Geometry check sheet. Reference: drawing and pictorial views, mm from the part's lowest x, y, z. Round coordinates to 2 decimals unless told otherwise and drop trailing zeros. Write each loop counter-clockwise with the first axis right and the second up, starting at its lowest first coordinate (ties: lowest second). Pieces come first, ordered by that corner, then holes. Notation, with made-up numbers: (78, -2) - (100, -2) arc R15 cw to (100, 13) - close; hole circle Ø10 at (88, -40). An arc over 180 degrees is marked (long way). Return JSON: item names as keys, results as strings.
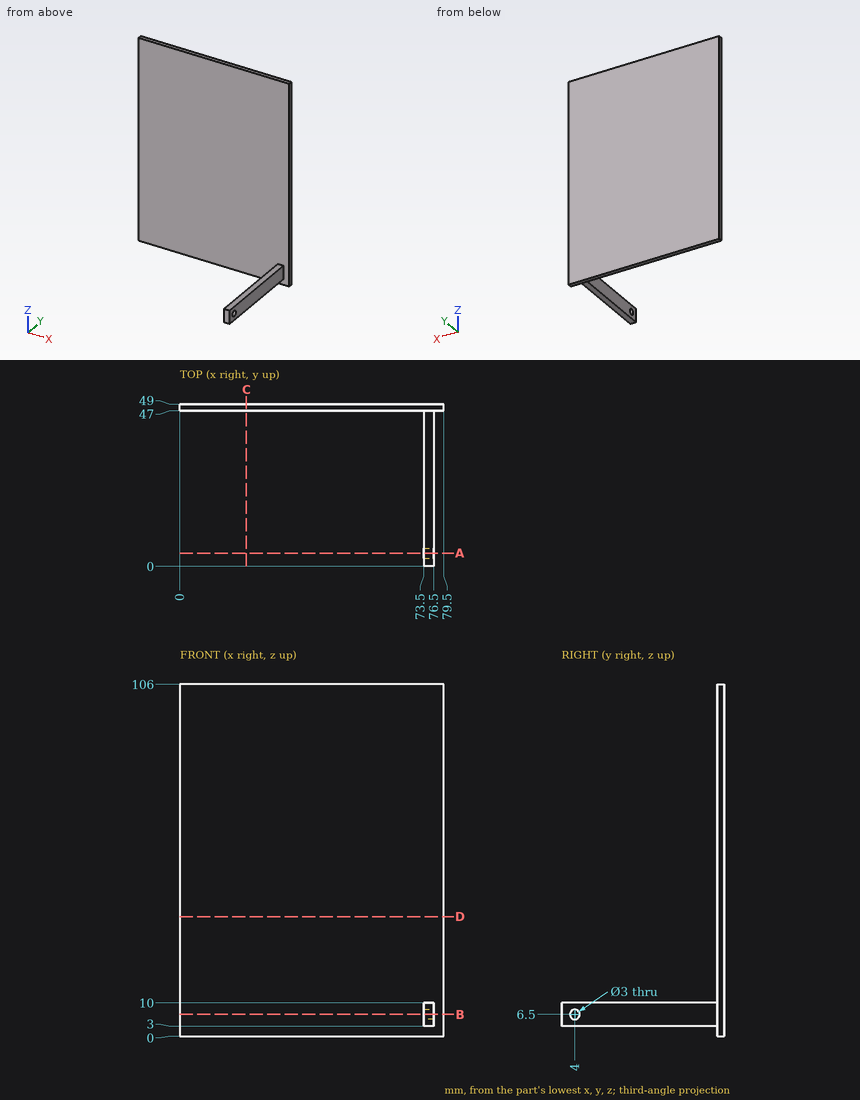
(1) Section check A-A, the plane y = 4. Enter the section's corners in (x, z), plus the area to 3 significant figures.
Response values:
{"outline": "(73.5, 3) - (76.5, 3) - (76.5, 5) - (73.5, 5) - close; (73.5, 8) - (76.5, 8) - (76.5, 10) - (73.5, 10) - close", "area": "12.0 mm^2"}
(2) Section check D-D, the plane z = 36. Enter the section's corners in (x, y).
Response values:
{"outline": "(0, 47) - (79.5, 47) - (79.5, 49) - (0, 49) - close"}
(3) Section check C-C, the plane x = 20. Enter the section's corners in (y, z), plus the area to 3 significant figures.
Response values:
{"outline": "(47, 0) - (49, 0) - (49, 106) - (47, 106) - close", "area": "212 mm^2"}
(4) Material ranges on line 1 along Y through (x, z) = (74.5, 6.5); line 2 along Y through (x, z) = (66.5, 35.5), recorded low to high. Write a range as [from, to].
Response values:
{"line 1": "y = [0, 2.5], [5.5, 49]", "line 2": "y = [47, 49]"}
(5) Gauge pin test, flat ends, axial feed: pin 1 (12 mm diameter, centred on x = 33.5, z = 71.5, fed in from -Y); pin 2 (7.5 mm diameter, centred on y = 27.5, z = 5.5, fed in from -X); pin 3 (3.5 mm diameter, centred on y = 20, z = 5.5, fed in from +X). Record the tip position at first contact, or that the pin passes through.
Response values:
{"pin 1": "stops at y = 47", "pin 2": "stops at x = 73.5", "pin 3": "stops at x = 76.5"}
(6) Section check B-B, the plane z = 6.5. Enter the section's corners in (x, y).
Response values:
{"outline": "(0, 47) - (73.5, 47) - (73.5, 5.5) - (76.5, 5.5) - (76.5, 47) - (79.5, 47) - (79.5, 49) - (0, 49) - close; (73.5, 0) - (76.5, 0) - (76.5, 2.5) - (73.5, 2.5) - close"}
